```python
from build123d import *

# Parameters (mm, degrees)
F0_R      = 50
F1_DEPTH  = 25
F2_R      = 52
F2_R_2    = 50
F3_DEPTH  = 10
F5_T      = -1.5
F6_R      = 33.5
F6_R_2    = 31.5
F7_DEPTH  = 5
F8_R      = 1
F9_R      = 32
F10_DEPTH = 25


# Not quite as in the source:
# - a feature of the source that left no trace in its solid (it failed there, or was rolled back) is left out


with BuildPart() as f1:
    # F0 (on Front) → F1 (new body)
    with BuildSketch(Plane.XZ):
        Circle(F0_R)
    extrude(amount=F1_DEPTH)

    # F2 (on face) → F3 (join)
    with BuildSketch(Plane.XZ.offset(25)):
        Circle(F2_R)
        Circle(F2_R_2, mode=Mode.SUBTRACT)
        Circle(F2_R_2)
    extrude(amount=F3_DEPTH)

    # F5
    f5_openings = [f1.faces().sort_by_distance(p)[0] for p in [
        (0, 0, 0),
    ]]
    offset(amount=F5_T, openings=f5_openings, kind=Kind.INTERSECTION)

    # F6 (on face) → F7 (join)
    with BuildSketch(Plane(origin=(0, -33.5, 0), x_dir=(-1, 0, 0), z_dir=(0, 1, 0))):
        Circle(F6_R)
        Circle(F6_R_2, mode=Mode.SUBTRACT)
    extrude(amount=F7_DEPTH)

    # F8
    f8_edges = [f1.edges().sort_by_distance(p)[0] for p in [
        (31.5, -28.5, 0),
        (-52, -35, 0),
        (-50, 0, 0),
    ]]
    fillet(f8_edges, radius=F8_R)

    # F9 (on face) → F10 (cut)
    with BuildSketch(Plane.XZ.offset(35)):
        Circle(F9_R)
    extrude(amount=-F10_DEPTH, mode=Mode.SUBTRACT)


solid = f1.part
```
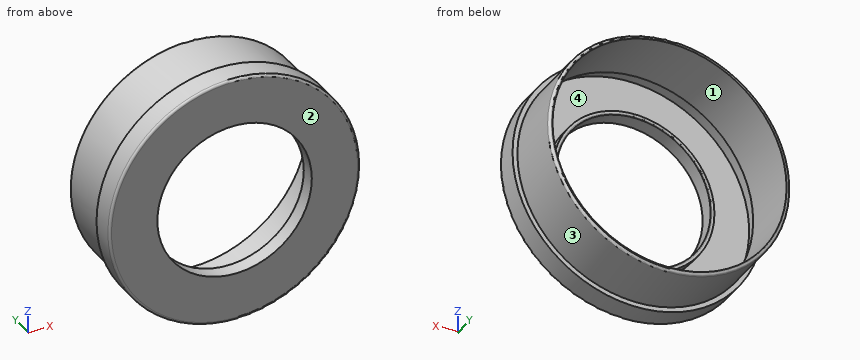
Check sheet for the modelled part. Datum: model origin and axes. Units: mm. Face numbers are marked on the shaded views. Give positions to 0.01 mm unless a question says otherwise; leave off trailing zeros. Order: outer loops, then holes, each group sorted by start corner. A loop starts at its lowest first (then second) coordinate and runs counter-clockwise, first axis right, second up. Notation, with made-up numbers: (1.5, 64) -> (36.5, 64) arc R18 cw to (36.5, 81) -> close; hole circle Ø1 at (20.5, 58). An arc over 180 degrees is marked (long way). Use CSV: the item, a comma, the result in double quotes. Start each with the question number.
1) Go/stop test with flat-tipped pins: P1, Ø8, axis at x = -17, z = -30, coming from the +Y side; P2, Ø5, axis at y = -17.5, z = -22.5, coming from the -X side; P3, Ø1, axis at y = -18.5, z = -41, coming from the -X side. Record where each tip stops, or that it passes through.
2) Sectioned sample at C-C, the plane y = -6. Record the boundary of the cut face in (x, z), plus the area to 3 significant figures.
3) Mould release check, pull along Z, two halves, no side actions. Record for the marked faces 1, 2, 3 and 4: released by +Z, released by -Z, zero draft, split by the parting line, or undercut.
4) Material ranges on line 1 (Z direction, x = 0, y = -32.75); line 2 (Z direction, x = 0, y = -28); line 3 (X direction, y = -31, z = 20), recorded low to high. Write a range as from..to.
Recorded:
1,P1,"y = -28.5"
1,P2,"x = -45.83"
1,P3,"x = -29.32"
2,outline,"circle Ø100 at (0, 0); hole circle Ø97 at (0, 0)"
2,area,"464 mm2"
3,face 1,"undercut"
3,face 2,"zero draft"
3,face 3,"split by the parting line"
3,face 4,"undercut"
4,line 1,"-52..-50.5, -33.5..-32, 32..33.5, 50.5..52"
4,line 2,"-52..-50.5, 50.5..52"
4,line 3,"-48..-46.37, -26.87..-24.98, 24.98..26.87, 46.37..48"
